from build123d import *

# Parameters (mm, degrees)
PAD_DEPTH    = 2
FILLET_R     = 4
FILLET001_R  = 6
POCKET_DEPTH = 5


with BuildPart() as part:
    # Sketch → Pad (new body)
    with BuildSketch(Plane.XY):
        Polygon((-115, 111), (115, 111), (110, -20), (-110, -20), align=None)
    extrude(amount=PAD_DEPTH)

    # Fillet
    fillet_edges = [part.edges().sort_by_distance(p)[0] for p in [
        (-110, -20, 1),
        (110, -20, 1),
    ]]
    fillet(fillet_edges, radius=FILLET_R)

    # Fillet001
    fillet001_edges = [part.edges().sort_by_distance(p)[0] for p in [
        (-115, 111, 1),
        (115, 111, 1),
    ]]
    fillet(fillet001_edges, radius=FILLET001_R)

    # Sketch001 (on Face5 of Fillet001) → Pocket (cut)
    with BuildSketch(Plane.XY.offset(2)):
        with BuildLine():
            Line((-88.5, 106), (88.5, 106))
            ThreePointArc((96.5, 98), (94.156854, 103.656854), (88.5, 106))
            Line((96.5, 98), (96.5, 3))
            ThreePointArc((88.5, -5), (94.156854, -2.656854), (96.5, 3))
            Line((88.5, -5), (-88.5, -5))
            ThreePointArc((-96.5, 3), (-94.156854, -2.656854), (-88.5, -5))
            Line((-96.5, 3), (-96.5, 98))
            ThreePointArc((-88.5, 106), (-94.156854, 103.656854), (-96.5, 98))
        make_face()
    extrude(amount=-POCKET_DEPTH, mode=Mode.SUBTRACT)


solid = part.part
Verification items for the finished model (mm, model axes). A direction names the side the tool comes from. Coordinates: 2 decimals unless noted, no trailing zeros. Order: outer loops, then holes, each group sorted by start corner. A loop starts at its lowest first (then second) coordinate and runs counter-clockwise, first axis right, second up. Notation, with made-up numbers: (1.25, 11.25) -> (7.25, 11.25) arc R19 ccw to (7.25, 23.25) -> close; hole circle Ø5 at (6, 64). An arc over 180 degrees is marked (long way). Put each result on its own line as item: value. Start each with the question number.
1. Material ranges on L1, parallel to Y at x = -85, z = 1.35; L2, parallel to X at y = 67, z = 0.55; L3, parallel to X at y = 5, z = 0.35, recorded low to high. Write a range as [from, to].
2. Mould release check, pull along Y, two halves, no side actions. Record for faces 3 (the cylindrical face through (94.219, 103.594, 1.014)), 4 (the flat face through (1, -8, 2)), 5 (the flat face through (112.487, 45.156, 0.986)), 6 (the cylindrical face through (-94.094, 103.719, 1.014)): released by +Y, released by -Y, zero draft, split by the parting line, or undercut.
3. Cross-section at C-C, the plane y = 52. Record the boundary of the cut face in (x, z), then the cut area to 3 significant figures.
4. Access from +Z, -Z, +X, -X, +Y, -Y to the whole of each face (thin tool, end or side, straight path). Record for faces 1 (the cylindrical face through (94.094, -2.719, 1.014)), 2 (the flat face through (-112.422, 43.463, 0.986)).
5. Cross-section at A-A, the plane x = -74.5. Record the boundary of the cut face in (y, z).
6. Cross-section at B-B, the plane z = 0.6. Record the boundary of the cut face in (x, y).
7. Go/stop test with flat-tipped pins: pin 1 Ø0.6 at (y, z) = (67, 1) entering from +X; pin 2 Ø0.6 at (y, z) = (32, 0.5) entering from -X. Record where each tip stops, or that it passes through.
Computed:
1. L1: [-20, -5], [106, 111]
1. L2: [-113.32, -96.5], [96.5, 113.32]
1. L3: [-110.95, -96.5], [96.5, 110.95]
2. face 3: undercut
2. face 4: zero draft
2. face 5: released by -Y
2. face 6: undercut
3. outline: (-112.75, 0) -> (-96.5, 0) -> (-96.5, 2) -> (-112.75, 2) -> close; (96.5, 0) -> (112.75, 0) -> (112.75, 2) -> (96.5, 2) -> close
3. area: 65.0 mm2
4. face 1: +Z, -Z
4. face 2: +Z, -Z, -X, -Y
5. outline: (-20, 0) -> (-5, 0) -> (-5, 2) -> (-20, 2) -> close; (106, 0) -> (111, 0) -> (111, 2) -> (106, 2) -> close
6. outline: (-114.76, 104.77) -> (-110.15, -16.15) arc R4 ccw to (-106.15, -20) -> (106.15, -20) arc R4 ccw to (110.15, -16.15) -> (114.76, 104.77) arc R6 ccw to (108.77, 111) -> (-108.77, 111) arc R6 ccw to start; hole (-96.5, 3) arc R8 ccw to (-88.5, -5) -> (88.5, -5) arc R8 ccw to (96.5, 3) -> (96.5, 98) arc R8 ccw to (88.5, 106) -> (-88.5, 106) arc R8 ccw to (-96.5, 98) -> close
7. pin 1: x = 113.33
7. pin 2: x = -112
